```python
from build123d import *

# Parameters (mm, degrees)
EXTRUDE_1_DEPTH     = 15
SKETCH_2_R          = 22.25
CUT_EXTRUDE_2_DEPTH = 60.213596412
FILLET_1_R          = 1


with BuildPart() as part:
    # 草图1 → 拉伸1 (new body)
    with BuildSketch(Plane.XY):
        Polygon((21.650635095, -37.5), (43.301270189, 0), (21.650635095, 37.5), (-21.650635095, 37.5), (-43.301270189, 0), (-21.650635095, -37.5), align=None)
    extrude(amount=EXTRUDE_1_DEPTH)

    # 草图2 → 拉伸2 (cut, through all)
    with BuildSketch(Plane.XY.offset(15)):
        Circle(SKETCH_2_R)
    extrude(amount=-CUT_EXTRUDE_2_DEPTH, mode=Mode.SUBTRACT)

    # 圆角1
    fillet_1_edges = [part.edges().sort_by_distance(p)[0] for p in [
        (32.475952642, 18.75, 15),
        (0, 37.5, 15),
        (-32.475952642, 18.75, 15),
        (-32.475952642, -18.75, 15),
        (-22.25, 0, 0),
        (-22.25, 0, 15),
        (0, -37.5, 15),
        (-32.475952642, -18.75, 0),
        (-32.475952642, 18.75, 0),
        (0, 37.5, 0),
        (32.475952642, -18.75, 15),
        (32.475952642, 18.75, 0),
        (32.475952642, -18.75, 0),
        (0, -37.5, 0),
    ]]
    fillet(fillet_1_edges, radius=FILLET_1_R)


solid = part.part
```
The model under review builds one solid part; all positions refer to its coordinate system, in mm. Coordinates: 2 decimals unless noted, no trailing zeros. Write each loop counter-clockwise with the first axis right and the second up, starting at its lowest first coordinate (ties: lowest second). Pieces come first, ordered by that corner, then holes. Notation, with made-up numbers: (-27.5, 22) - (14.5, 22) arc R21 ccw to (14.5, 39) - close; hole circle Ø3 at (-25, 41.25). An arc over 180 degrees is marked (long way). Write item = value, one per line.
(1) Mouldability with a two-part tool opening along Y and no side actions: class faces 1 (the face through (-32.628, -18.488, 7.409)), 2 (the face through (-16.399, 15.038, 7.591)), 3 (the face through (-32.37, 18.34, 14.71)), 4 (the face through (18, 17, 15)) as pulls with the +Y half, pulls with the -Y half, needs draft (parallel to the pull), parting line crosses it, or undercut.
Result sheet:
face_1 = pulls with the -Y half
face_2 = undercut
face_3 = pulls with the +Y half
face_4 = needs draft
(2) Consider section B-B, the plane x = 0. Give the boundary of the cut face in (y, z), then the cut area to 3 significant figures.
Result sheet:
outline = (-37.5, 1) arc R1 ccw to (-36.5, 0) - (-23.25, 0) arc R1 ccw to (-22.25, 1) - (-22.25, 14) arc R1 ccw to (-23.25, 15) - (-36.5, 15) arc R1 ccw to (-37.5, 14) - close; (22.25, 1) arc R1 ccw to (23.25, 0) - (36.5, 0) arc R1 ccw to (37.5, 1) - (37.5, 14) arc R1 ccw to (36.5, 15) - (23.25, 15) arc R1 ccw to (22.25, 14) - close
area = 456 mm^2
(3) Consider section A-A, the plane z = 4.75. Give the boundary of the cut face in (x, y), then the cut area to 3 significant figures.
Result sheet:
outline = (-43.3, 0) - (-21.65, -37.5) - (21.65, -37.5) - (43.3, 0) - (21.65, 37.5) - (-21.65, 37.5) - close; hole circle Ø44.5 at (0, 0)
area = 3,320 mm^2
(4) For line 1 (Y direction, x = 0, z = 6.5); line 2 (X direction, y = 18, z = 0.5); line 3 (Y direction, x = 6.5, z = 14), list the stretches that pass through material, from the lowest coordinate up. Write a range as [from, to].
Result sheet:
line_1 = [-37.5, -22.25], [22.25, 37.5]
line_2 = [-32.75, -13.31], [13.31, 32.75]
line_3 = [-37.5, -21.28], [21.28, 37.5]
(5) For P1, Ø4, axis at x = -28, z = 6.5, coming from the -Y side; P2, Ø8, axis at x = 29.5, z = 5.5, coming from the -Y side; P3, Ø2, axis at y = -22, z = 11.5, coming from the +X side, all flat-tipped, find the tip position at first contact; note any pin that passes through.
Result sheet:
P1 = -29.97
P2 = -30.83
P3 = 31.18
